```python
from build123d import *

# Parameters (mm, degrees)
SKETCH1_R           = 20
BOSS_EXTRUDE1_DEPTH = 25.8
SKETCH2_R           = 1.5
BOSS_EXTRUDE4_DEPTH = 2
CHAMFER1_SIZE       = 1
SKETCH3_R           = 20
SKETCH3_R_2         = 15
BOSS_EXTRUDE5_DEPTH = 3


with BuildPart() as part:
    # Sketch1 → Boss-Extrude1 (new body)
    with BuildSketch(Plane(origin=(0, 0, 0), x_dir=(1, 0, 0), z_dir=(0, 1, 0))):
        with Locations(Location((0, 0, 0), (0, 0, 90))):
            Circle(SKETCH1_R)
    extrude(amount=BOSS_EXTRUDE1_DEPTH)

    # Sketch2 → Boss-Extrude4 (add)
    # profile 1 of 4: a face of its own
    with BuildSketch(Plane(origin=(0, 0, 0), x_dir=(1, 0, 0), z_dir=(0, 1, 0))):
        with BuildLine():
            Line((-12.348666302, 15.732464542), (-16.053266193, 20.452203904))
            ThreePointArc((-16.053266193, 20.452203904), (-18.426104242, 18.343355267), (-20.524251517, 15.961049453))
            Line((-20.524251517, 15.961049453), (-15.787885783, 12.277730349))
            ThreePointArc((-15.787885783, 12.277730349), (-14.17392634, 14.110273282), (-12.348666302, 15.732464542))
        make_face()
        with Locations(Location((-16.300015291, 16.226814275, 0), (0, 0, 270))):
            Circle(SKETCH2_R, mode=Mode.SUBTRACT)
    # profile 2 of 4: a face of its own
    with BuildSketch(Plane(origin=(0, 0, 0), x_dir=(1, 0, 0), z_dir=(0, 1, 0))):
        with BuildLine():
            Line((15.732464542, 12.348666302), (20.452203904, 16.053266193))
            ThreePointArc((20.452203904, 16.053266193), (18.343355267, 18.426104242), (15.961049453, 20.524251517))
            Line((15.961049453, 20.524251517), (12.277730349, 15.787885783))
            ThreePointArc((12.277730349, 15.787885783), (14.110273282, 14.17392634), (15.732464542, 12.348666302))
        make_face()
        with Locations(Location((16.226814275, 16.300015291, 0), (0, 0, 270))):
            Circle(SKETCH2_R, mode=Mode.SUBTRACT)
    # profile 3 of 4: a face of its own
    with BuildSketch(Plane(origin=(0, 0, 0), x_dir=(1, 0, 0), z_dir=(0, 1, 0))):
        with BuildLine():
            Line((12.348666302, -15.732464542), (16.053266193, -20.452203904))
            ThreePointArc((16.053266193, -20.452203904), (18.426104242, -18.343355267), (20.524251517, -15.961049453))
            Line((20.524251517, -15.961049453), (15.787885783, -12.277730349))
            ThreePointArc((15.787885783, -12.277730349), (14.17392634, -14.110273282), (12.348666302, -15.732464542))
        make_face()
        with Locations(Location((16.300015291, -16.226814275, 0), (0, 0, 270))):
            Circle(SKETCH2_R, mode=Mode.SUBTRACT)
    # profile 4 of 4: a face of its own
    with BuildSketch(Plane(origin=(0, 0, 0), x_dir=(1, 0, 0), z_dir=(0, 1, 0))):
        with BuildLine():
            Line((-15.732464542, -12.348666302), (-20.452203904, -16.053266193))
            ThreePointArc((-20.452203904, -16.053266193), (-18.343355267, -18.426104242), (-15.961049453, -20.524251517))
            Line((-15.961049453, -20.524251517), (-12.277730349, -15.787885783))
            ThreePointArc((-12.277730349, -15.787885783), (-14.110273282, -14.17392634), (-15.732464542, -12.348666302))
        make_face()
        with Locations(Location((-16.226814275, -16.300015291, 0), (0, 0, 270))):
            Circle(SKETCH2_R, mode=Mode.SUBTRACT)
    extrude(amount=BOSS_EXTRUDE4_DEPTH)

    # Chamfer1
    # the kernel refuses this chamfer: 1 mm, written as the material it takes off along each edge
    with BuildSketch(Plane(origin=(-20.452203904, -2.571682988, 16.053266193), x_dir=(0.786623227084006, 0, -0.6174333151134171), z_dir=(0, 1, 0)), Plane(origin=(16.053266193, -2.571682988, 20.452203904), x_dir=(-0.6174333151134189, 0, -0.7866232270840047), z_dir=(0, 1, 0)), Plane(origin=(20.452203904, -2.571682988, -16.053266193), x_dir=(-0.7866232270840033, 0, 0.6174333151134205), z_dir=(0, 1, 0)), Plane(origin=(-16.053266193, -2.571682988, -20.452203904), x_dir=(0.6174333151134251, 0, 0.7866232270839999), z_dir=(0, 1, 0))) as chamfer1_piece_1:
        with BuildLine():
            Line((CHAMFER1_SIZE, 0), (0.018531237, -0.981468763))
            ThreePointArc((0.018531237, -0.981468763), (0.004898706, -0.504686734), (0, 0))
            Line((0, 0), (CHAMFER1_SIZE, 0))
        make_face()
    extrude(amount=7.143365976, mode=Mode.SUBTRACT)
    with BuildSketch(Plane(origin=(-15.961049453, -2.571682988, 20.524251517), x_dir=(0.6138865174304216, 0, -0.7893942891338579), z_dir=(0, 1, 0)), Plane(origin=(20.524251517, -2.571682988, 15.961049453), x_dir=(-0.7893942891338613, 0, -0.6138865174304171), z_dir=(0, 1, 0)), Plane(origin=(15.961049453, -2.571682988, -20.524251517), x_dir=(-0.6138865174304153, 0, 0.7893942891338627), z_dir=(0, 1, 0)), Plane(origin=(-20.524251517, -2.571682988, -15.961049453), x_dir=(0.7893942891338679, 0, 0.6138865174304086), z_dir=(0, 1, 0))) as chamfer1_piece_2:
        with BuildLine():
            Line((CHAMFER1_SIZE, 0), (0.018531237, 0.981468763))
            ThreePointArc((0.018531237, 0.981468763), (0.004898706, 0.504686734), (0, 0))
            Line((0, 0), (CHAMFER1_SIZE, 0))
        make_face()
    extrude(amount=7.143365976, mode=Mode.SUBTRACT)

    # Sketch3 → Boss-Extrude5 (add)
    with BuildSketch(Plane(origin=(0, 25.8, 0), x_dir=(1, 0, 0), z_dir=(0, 1, 0))):
        with Locations(Location((0, 0, 0), (0, 0, 52.128942853))):
            Circle(SKETCH3_R)
        with Locations(Location((0, 0, 0), (0, 0, 270))):
            Circle(SKETCH3_R_2, mode=Mode.SUBTRACT)
    extrude(amount=BOSS_EXTRUDE5_DEPTH)


solid = part.part
```
Build history of the part. All positions in model axes, mm. A direction names the side the tool comes from. Coordinates: 2 decimals unless noted, no trailing zeros. Order: outer loops, then holes, each group sorted by start corner. A loop starts at its lowest first (then second) coordinate and runs counter-clockwise, first axis right, second up. Notation, with made-up numbers: M 51,33 L 87,33 A9 cw 87,47 Z; hole C 7,-3 d5. An arc over 180 degrees is marked long. One line per question, with ' | ' between items. Start each with the question number.
1. Wall check: line 1 along Y through (x, z) = (9, 8); line 2 along Z through (x, y) = (2, 12.75); line 3 along Y through (x, z) = (-16.5, 18). Give the ranges that are in metal, low to high. Write a range as [from, to].
2. Mould opens along X. For faces 6 (the face through (-17.67, 0.99, 13.87)), 7 (the face through (-13.87, 0.99, -17.67)), 8 (the face through (17.67, 0.99, -13.87)) say: +X half, -X half, draft (parallel to the pull), parting line (faces both ways), or undercut.
3. Flat gauge pins, fed straight in: P1, Ø2.5, axis at x = 16.23, z = -16.3, coming from the -Y side; P2, Ø2, axis at y = 3.5, z = -5, coming from the +X side; P3, Ø8, axis at y = 17, z = 1.5, coming from the -X side; P4, Ø9, axis at x = 1.5, z = 1, coming from the +Y side. Where does each tip first touch, or does it go through?
4. Cut at B-B (z = 0). Write the cut outline in (x, y), plus the area to 3 significant figures.
5. Cut at D-D (x = -14). Write the cut outline in (y, z).
6. Cut at C-C (y = 23.75). Write the cut outline in (x, z).
7. Cut at A-A (x = 0). Write the cut outline in (y, z), plus the area to 3 significant figures.
8. Tool access for faces 1 (the face through (13.87, 0.99, 17.67)), 2 (the face through (18, 1, 14)), 3 (the face through (-19.82, 0.99, -16.03)), 4 (the face through (0, 25.8, 0)), 5 (the face through (15, 2, 15)): list every direction of +Z, -Z, +X, -X, +Y, -Y with a clear straight run to the whole face (end or side of a thin tool).
The answers:
1) line 1: y = [0, 25.8] | line 2: z = [-19.9, 19.9] | line 3: y = [0, 2]
2) face 6: -X half | face 7: undercut | face 8: +X half
3) P1: passes through | P2: stops at x = 19.6 | P3: stops at x = -20 | P4: stops at y = 25.8
4) outline: M -20,0 L 20,0 L 20,28.8 L 15,28.8 L 15,25.8 L -15,25.8 L -15,28.8 L -20,28.8 Z | area: 1,060 mm2
5) outline: M 0,-17.84 L 2,-17.84 L 2,-14.28 L 28.8,-14.28 L 28.8,-5.39 L 25.8,-5.39 L 25.8,5.39 L 28.8,5.39 L 28.8,14.28 L 2,14.28 L 2,18 L 0,18 Z
6) outline: C 0,0 d40
7) outline: M 0,-20 L 28.8,-20 L 28.8,-15 L 25.8,-15 L 25.8,15 L 28.8,15 L 28.8,20 L 0,20 Z | area: 1,060 mm2
8) face 1: +Z, +Y, -Y | face 2: +X, +Y, -Y | face 3: -X, +Y, -Y | face 4: +Y | face 5: +Z, +X, +Y
